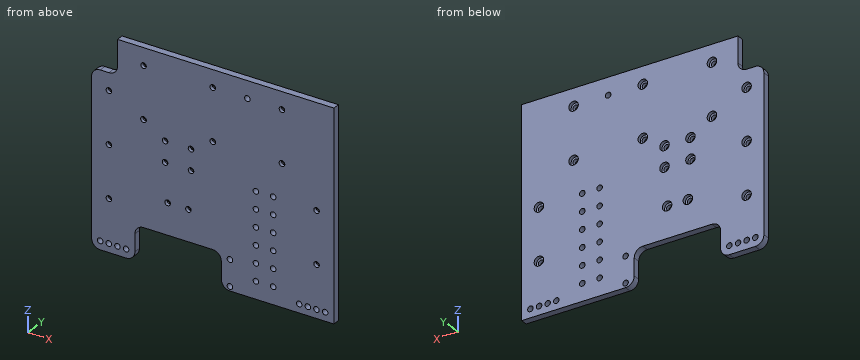
Autodesk Inventor part; units mm, degrees
ref_plane "YZ Plane" through (0, 0, 0) normal (1, 0, 0) x (0, 1, 0)
ref_plane "XZ Plane" through (0, 0, 0) normal (0, 1, 0) x (-1, 0, 0)
ref_plane "XY Plane" through (0, 0, 0) normal (0, 0, 1) x (1, 0, 0)
sketch "Sketch1" plane through (0, 0, 0) normal (0, 1, 0) x (-1, 0, 0)
  circle A0 centre (51.9082, -238.2442) radius 1.6
  circle A1 centre (46.9082, -238.2442) radius 1.6
  line L0 (41.8423, -223.2442) -> (41.8423, -243.2442)
  line L1 (41.8423, -243.2442) -> (-8.0918, -243.2442)
  line L2 (-8.0918, -223.2442) -> (41.8423, -223.2442)
  line L3 (-8.0918, -243.2442) -> (-8.0918, -223.2442)
  circle A2 centre (56.9082, -238.2442) radius 1.6
  circle A3 centre (61.9082, -238.2442) radius 1.6
  circle A4 centre (9.4082, -171.2442) radius 2.75
  line L4 (66.8423, -243.2442) -> (-73.1577, -243.2442)
  line L5 (66.8423, -123.2442) -> (66.8423, -243.2442)
  line L6 (-3.1577, -123.2442) -> (-3.1577, -243.2442) construction
  line L7 (71.8423, -183.2442) -> (-68.1577, -183.2442) construction
  line L8 (-73.1577, -123.2442) -> (66.8423, -123.2442)
  line L9 (-73.1577, -243.2442) -> (-73.1577, -123.2442)
  circle A5 centre (-63.1577, -213.2442) radius 1.6
  circle A6 centre (-63.1577, -183.2442) radius 1.6
  circle A7 centre (-63.1577, -183.2442) radius 2.75
  circle A8 centre (-63.1577, -213.2442) radius 2.75
  circle A9 centre (-68.0918, -238.2442) radius 1.6
  circle A10 centre (-63.0918, -238.2442) radius 1.6
  circle A11 centre (-58.0918, -238.2442) radius 1.6
  circle A12 centre (-53.0918, -238.2442) radius 1.6
  circle A13 centre (9.4082, -171.2442) radius 1.6
  circle A14 centre (24.4082, -171.2442) radius 1.6
  circle A15 centre (24.4082, -171.2442) radius 2.75
  circle A16 centre (9.4082, -183.2442) radius 1.6
  circle A17 centre (9.4082, -183.2442) radius 2.75
  circle A18 centre (24.4082, -183.2442) radius 1.6
  circle A19 centre (24.4082, -183.2442) radius 2.75
  circle A20 centre (10.9082, -205.2442) radius 1.6
  circle A21 centre (10.9082, -205.2442) radius 2.75
  circle A22 centre (22.9082, -205.2442) radius 1.6
  circle A23 centre (22.9082, -205.2442) radius 2.75
  circle A24 centre (-43.1577, -133.2442) radius 1.6
  circle A25 centre (-43.1577, -133.2442) radius 2.75
  circle A26 centre (-3.1577, -133.2442) radius 1.6
  circle A27 centre (-3.1577, -133.2442) radius 2.75
  circle A28 centre (36.8423, -133.2442) radius 1.6
  circle A29 centre (36.8423, -133.2442) radius 2.75
  circle A30 centre (56.9082, -128.2442) radius 1.6
  circle A31 centre (61.9082, -128.2442) radius 1.6
  circle A32 centre (56.8423, -213.2442) radius 1.6
  circle A33 centre (56.8423, -213.2442) radius 2.75
  circle A34 centre (56.8423, -183.2442) radius 1.6
  circle A35 centre (56.8423, -183.2442) radius 2.75
  circle A36 centre (56.8423, -153.2442) radius 1.6
  circle A37 centre (56.8423, -153.2442) radius 2.75
  circle A38 centre (-13.0918, -240.7442) radius 1.6
  circle A39 centre (-13.0918, -225.7442) radius 1.6
  circle A40 centre (-38.0918, -233.2442) radius 1.6
  circle A41 centre (-28.0918, -233.2442) radius 1.6
  circle A42 centre (-28.0918, -223.2442) radius 1.6
  circle A43 centre (-38.0918, -223.2442) radius 1.6
  circle A44 centre (-28.0918, -203.2442) radius 1.6
  circle A45 centre (-28.0918, -213.2442) radius 1.6
  circle A46 centre (-38.0918, -203.2442) radius 1.6
  circle A47 centre (-38.0918, -213.2442) radius 1.6
  line L10 (-33.0918, -198.2442) -> (-28.0918, -198.2442)
  circle A48 centre (-28.0918, -183.2442) radius 1.6
  circle A49 centre (-38.0918, -183.2442) radius 1.6
  circle A50 centre (-38.0918, -193.2442) radius 1.6
  circle A51 centre (-28.0918, -193.2442) radius 1.6
  circle A52 centre (36.8423, -163.2442) radius 1.65
  circle A53 centre (36.8423, -163.2442) radius 2.75
  circle A54 centre (-3.1577, -163.2442) radius 1.65
  circle A55 centre (-3.1577, -163.2442) radius 2.75
  circle A56 centre (-43.1577, -163.2442) radius 1.65
  circle A57 centre (-43.1577, -163.2442) radius 2.75
  line L11 (66.8423, -123.2442) -> (51.8423, -123.2442)
  line L12 (51.8423, -123.2442) -> (51.8423, -143.2442)
  line L13 (51.8423, -143.2442) -> (66.8423, -143.2442)
  line L14 (66.8423, -143.2442) -> (66.8423, -123.2442)
  circle A58 centre (-23.1577, -133.2442) radius 1.6
  point P0 (0, -190.5)
  point P1 (16.9082, -168.6317)
  point P2 (16.9082, -205.2442)
  dimension "d33" = 140
  dimension "d34" = 120
  dimension "d35" = 10
  dimension "d36" = 10
  dimension "d37" = 10
  dimension "d39" = 10
  dimension "d40" = 10
  dimension "d41" = 10
  dimension "d42" = 10
  dimension "d43" = 10
  dimension "d44" = 40
  dimension "d45" = 40
  dimension "d46" = 3.2
  dimension "d47" = 2.5
  dimension "d48" = 5
  dimension "d49" = 3.2
  dimension "d50" = 15
  dimension "d60" = 3.2
  dimension "d61" = 3.2
  dimension "d63" = 3.2
  dimension "d65" = 3.2
  dimension "d66" = 10
  dimension "d69" = 10
  dimension "d70" = 10
  dimension "d71" = 10
  dimension "d76" = 3.3
  dimension "d77" = 5.5
  dimension "d78" = 30
  dimension "d79" = 3.3
  dimension "d80" = 5.5
  dimension "d81" = 15
  dimension "d82" = 20
  dimension "d84" = 3.2
  dimension "d85" = 20
extrude "Extrusion1" add sketch "Sketch1" along normal blind 4 contours L2 L3 L4 L9 L8 L12 L13 L5 L0
sketch "Sketch2" plane through (0, 4, 0) normal (0, 1, 0) x (1, 0, 0)
  point P0 (0, 0)
extrude "Extrusion2" add sketch "Sketch1" along normal blind 2 contours L2 L3 L4 L9 L8 L12 L13 L5 L0 | A4 | A7 | A8 | A15 | A17 | A19 | A21 | A23 | A25 | A27 | A29 | A33 | A35 | A37 | A53 | A55 | A57
fillet "Fillet1" radius 5 7 edges at (-51.8423, 2, -143.2442) (-66.8423, 2, -143.2442) (-66.8423, 2, -243.2442) (8.0918, 2, -243.2442) (8.0918, 2, -223.2442) (-41.8423, 2, -223.2442) (-41.8423, 2, -243.2442)
properties part number "Fix Casis Kanan Depan_3DPrint"
CAD build for the part. Positions are in the model's coordinates, mm. Give positions to 0.01 mm unless a question says otherwise; leave off trailing zeros.
(1) Flat gauge pins, fed straight in: pin 1 (6 mm diameter, centred on x = -56, z = -212.5, fed in from +Y); pin 2 (4.5 mm diameter, centred on x = -56.84, z = -213.24, fed in from +Y). Where does each tip first touch, or does it go through?
(2) Saw through at A-A, the plane y = 1.3. State how many separate pieces and enclosed holes the cut face has, then the cut area to 3 significant figures.
(3) Drill centre lines: L1, parallel to X at y = 2.25, z = -213; L2, parallel to X at y = 3.15, z = -205; L3, parallel to X at y = 3.5, z = -151. Where is each one in solid material? Low to high.
Results found:
1. pin 1: stops at y = 4
1. pin 2: stops at y = 2
2. separate pieces: 1
2. enclosed holes: 40
2. area: 15,200 mm2
3. L1: x = -66.84 to -59.58, -54.1 to 26.51, 29.67 to 36.51, 39.67 to 60.42, 65.9 to 73.16
3. L2: x = -66.84 to -25.65, -20.17 to -13.65, -8.17 to 73.16
3. L3: x = -66.84 to -58.43, -55.25 to 73.16
